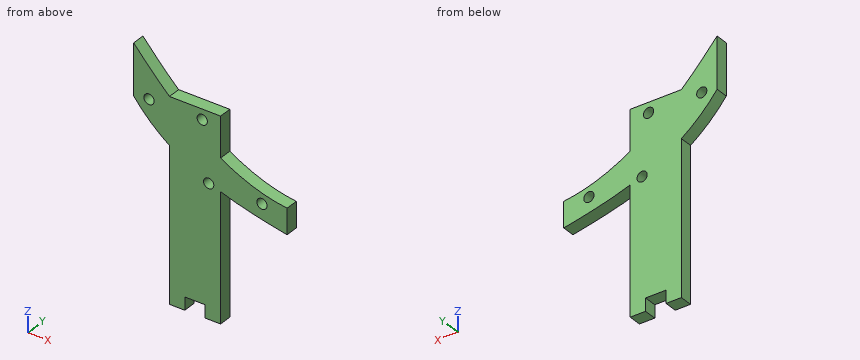
```python
from build123d import *

# Parameters (mm, degrees)
F1_DEPTH  = 3.175
F2_W      = 12.7
F2_H      = 39.6141249724
F3_DEPTH  = 3.175
F5_DEPTH  = 3.175
F6_R      = 1.27
F7_DEPTH  = 3.1760001
F8_R      = 1.27
F9_DEPTH  = 3.1760001
F10_W     = 5.08
F10_H     = 6.35
F11_DEPTH = 25.4


with BuildPart() as f1:
    # F0 (on Front) → F1 (new body)
    with BuildSketch(Plane.XZ):
        with BuildLine():
            add(Edge.make_bspline(
                [(-38.1, 19.05), (-28.3741913736, 6.3939620741), (-14.1141656786, 2.7637183666), (0, 0)],
                knots=[0, 0, 0, 0, 42.5970949714, 42.5970949714, 42.5970949714, 42.5970949714], degree=3))
            Line((0, 0), (0, 6.35))
            add(Edge.make_bspline(
                [(-38.1, 31.75), (-29.2279217392, 21.5179808438), (-16.6689809412, 8.3035267889), (0, 6.35)],
                knots=[0, 0, 0, 0, 45.7905011984, 45.7905011984, 45.7905011984, 45.7905011984], degree=3))
            Line((-38.1, 31.75), (-38.1, 19.05))
        make_face()
    extrude(amount=F1_DEPTH)

    # F2 (on face) → F3 (join, through all)
    with BuildSketch(Plane.XZ.offset(3.175)):
        with Locations((-22.8709825013, -7.5756740422)):
            Rectangle(F2_W, F2_H)
    extrude(amount=-F3_DEPTH)

    # F4 (on face) → F5 (join, through all)
    with BuildSketch(Plane.XZ.offset(3.175)):
        with BuildLine():
            Line((-16.5209825013, 22.2295189018), (-29.2209825013, 22.2295189018))
            add(Edge.make_bspline(
                [(-16.5209825013, 12.2313884441), (-21.2089143391, 15.0429542082), (-25.4366525194, 18.5639866867), (-29.2209825013, 22.2295189018)],
                knots=[45.7905011984, 45.7905011984, 45.7905011984, 45.7905011984, 61.4068288598, 61.4068288598, 61.4068288598, 61.4068288598], degree=3))
            Line((-16.5209825013, 12.2313884441), (-16.5209825013, 22.2295189018))
        make_face()
    extrude(amount=-F5_DEPTH)

    # F6 (on face) → F7 (cut, through all)
    with BuildSketch(Plane.XZ.offset(3.175)):
        with Locations((-34.29, 19.6895189018)):
            Circle(F6_R)
        with Locations((-21.082, 19.6895189018)):
            Circle(F6_R)
    extrude(amount=-F7_DEPTH, mode=Mode.SUBTRACT)

    # F8 (on face) → F9 (cut, through all)
    with BuildSketch(Plane.XZ.offset(3.175)):
        with Locations((-19.4714572281, 5.08)):
            Circle(F8_R)
        with Locations((-6.2634572281, 5.08)):
            Circle(F8_R)
    extrude(amount=-F9_DEPTH, mode=Mode.SUBTRACT)

    # F10 (on face) → F11 (cut)
    with BuildSketch(Plane.XZ.offset(3.175)):
        with Locations((-22.8709825013, -27.3827365284)):
            Rectangle(F10_W, F10_H)
    extrude(amount=-F11_DEPTH, mode=Mode.SUBTRACT)


solid = f1.part
```
Geometry: final body of the model. Coordinates: model frame, mm. Round coordinates to 2 decimals unless told otherwise and drop trailing zeros. Loops run counter-clockwise (first coordinate to the right, second up) from the corner with the lowest first, then second, coordinate; pieces in that order, holes last. Notation, with made-up numbers: (50, -29.5) -> (66, -29.5) arc R18 ccw to (66, -7.5) -> close; hole circle Ø8 at (-34.75, 47). An arc over 180 degrees is marked (long way). Use one line per item in the form item = value.
Item 1: Cut plane A-A on z = 5.08. Output: boundary loops of the cut face in (x, y) (3 decimals), then the cut area to 3 significant figures.
Evaluation:
outline = (-29.221, -3.175) -> (-20.741, -3.175) -> (-20.741, 0) -> (-29.221, 0) -> close; (-18.201, -3.175) -> (-7.533, -3.175) -> (-7.533, 0) -> (-18.201, 0) -> close; (-4.993, -3.175) -> (0, -3.175) -> (0, 0) -> (-4.993, 0) -> close
area = 76.6 mm2
Item 2: Material intervals for probe 1 along X at (y, z) = (-0.15, -1.5); probe 2 along Z at (x, y) = (-29, -2.9); probe 3 along X at (y, z) = (-1.05, 19), sorted ascending.
Evaluation:
probe_1 = -29.22 to -16.52
probe_2 = -27.38 to 22.23
probe_3 = -38.06 to -35.36, -33.22 to -22.15, -20.02 to -16.52
Item 3: Contact query for flat-ended pins moving along their axis: pin 1 Ø1.6 at (x, y) = (-23.5, -1) entering from -Z; pin 2 Ø1 at (x, y) = (-22, -2) entering from +Z; pin 3 Ø1.6 at (y, z) = (-2, -4) entering from +X. Output: stop coordinate, or through.
Evaluation:
pin_1 = -24.21
pin_2 = 22.23
pin_3 = -16.52
Item 4: Cut plane B-B on y = -2.2. Give the number of separate pieces and of enclosed holes in the cut face, then the cut area to 3 significant figures.
Evaluation:
separate_pieces = 1
enclosed_holes = 4
area = 816 mm2
Item 5: Cut plane C-C on z = -23. Output: boundary loops of the cut face in (x, y) (3 decimals).
Evaluation:
outline = (-29.221, -3.175) -> (-16.521, -3.175) -> (-16.521, 0) -> (-29.221, 0) -> close
